from build123d import *

# Parameters (mm, degrees)
F0_W     = 80
F0_H     = 80
F1_DEPTH = 10
F2_SIZE2 = 9.99999
F2_SIZE  = 9.99999
F3_W     = 10
F3_H     = 40
F4_DEPTH = 10
F6_DEPTH = 8


# Not quite as in the source:
# - a fillet or chamfer is up to 0.001 mm smaller than in the source, because OpenCascade refuses the exact size


with BuildPart() as f1:
    # F0 (on Top) → F1 (new body)
    with BuildSketch(Plane.XY):
        Rectangle(F0_W, F0_H)
    extrude(amount=F1_DEPTH)

    # F2 (size 10 and 10 in the source; OpenCascade refuses exactly that, so slightly less here)
    f2_edges = [f1.edges().sort_by_distance(p)[0] for p in [
        (0, 40, 10),
        (-40, 0, 10),
        (0, -40, 10),
        (40, 0, 10),
    ]]
    chamfer(f2_edges, length=F2_SIZE, length2=F2_SIZE2)

    # F3 (on face) → F4 (join)
    with BuildSketch(Plane.XY.offset(10)):
        with Locations((25, 0)):
            Rectangle(F3_W, F3_H)
        with Locations((-25, 0)):
            Rectangle(F3_W, F3_H)
    extrude(amount=F4_DEPTH)

    # F5 (on face) → F6 (cut)
    with BuildSketch(Plane.XY.offset(10)):
        with BuildLine():
            Line((-3.8890872965, -3.8890872965), (-10.2530483272, -10.2530483272))
            ThreePointArc((-10.2530483272, -10.2530483272), (-5.3489923662, -11.2285257082), (-2.5710678119, -7.0710678119))
            ThreePointArc((-2.5710678119, -7.0710678119), (-2.9136099156, -5.3489923662), (-3.8890872965, -3.8890872965))
        make_face()
        with BuildLine():
            Line((3.8890872965, 3.8890872965), (10.2530483272, 10.2530483272))
            ThreePointArc((10.2530483272, 10.2530483272), (3.8890872965, 10.2530483272), (3.8890872965, 3.8890872965))
        make_face()
        with BuildLine():
            ThreePointArc((-2.5710678119, 7.0710678119), (-5.3489923662, 11.2285257082), (-10.2530483272, 10.2530483272))
            Line((-10.2530483272, 10.2530483272), (-3.8890872965, 3.8890872965))
            ThreePointArc((-3.8890872965, 3.8890872965), (-2.9136099156, 5.3489923662), (-2.5710678119, 7.0710678119))
        make_face()
        with BuildLine():
            ThreePointArc((11.5710678119, 7.0710678119), (11.2285257082, 8.7931432575), (10.2530483272, 10.2530483272))
            Line((10.2530483272, 10.2530483272), (3.8890872965, 3.8890872965))
            ThreePointArc((3.8890872965, 3.8890872965), (8.7931432575, 2.9136099156), (11.5710678119, 7.0710678119))
        make_face()
        with BuildLine():
            ThreePointArc((3.8890872965, -3.8890872965), (3.8890872965, -10.2530483272), (10.2530483272, -10.2530483272))
            Line((10.2530483272, -10.2530483272), (3.8890872965, -3.8890872965))
        make_face()
        with BuildLine():
            Line((-3.8890872965, 3.8890872965), (-10.2530483272, 10.2530483272))
            ThreePointArc((-10.2530483272, 10.2530483272), (-10.2530483272, 3.8890872965), (-3.8890872965, 3.8890872965))
        make_face()
        with BuildLine():
            ThreePointArc((-3.8890872965, -3.8890872965), (-10.2530483272, -3.8890872965), (-10.2530483272, -10.2530483272))
            Line((-10.2530483272, -10.2530483272), (-3.8890872965, -3.8890872965))
        make_face()
        with BuildLine():
            Line((3.8890872965, -3.8890872965), (10.2530483272, -10.2530483272))
            ThreePointArc((10.2530483272, -10.2530483272), (11.2285257082, -8.7931432575), (11.5710678119, -7.0710678119))
            ThreePointArc((11.5710678119, -7.0710678119), (8.7931432575, -2.9136099156), (3.8890872965, -3.8890872965))
        make_face()
    extrude(amount=-F6_DEPTH, mode=Mode.SUBTRACT)


solid = f1.part
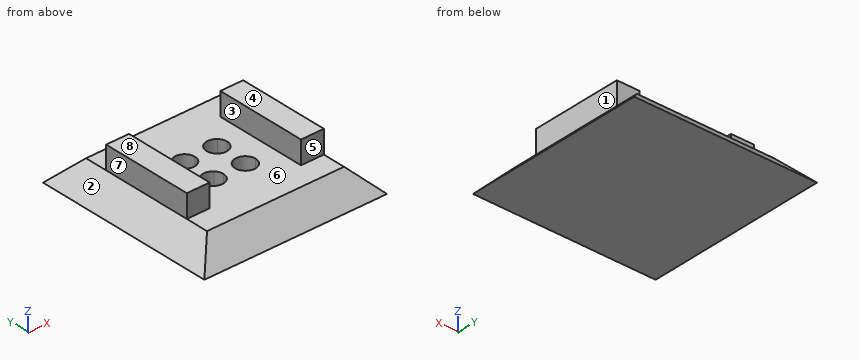
The listing builds one solid part. Answer for the finished solid, in the listing's coordinates (mm). Face numbers are marked on the shaded views. A direction names the side the tool comes from. Coordinates: 2 decimals unless noted, no trailing zeros. Order: outer loops, then holes, each group sorted by start corner. A loop starts at its lowest first (then second) coordinate and runs counter-clockwise, first axis right, second up. Notation, with made-up numbers: (62.25, 85) -> (78.25, 85) arc R27 ccw to (78.25, 114) -> close; hole circle Ø11 at (74.25, -29.5). An arc over 180 degrees is marked (long way). Answer in a Markdown table with one row per item. Add a question column.
Item 1: Determine the mould class of the marked faces 6, 7 and 8 for opening direction X: +X half, -X half, draft (parallel to the pull), parting line (faces both ways), or undercut.
Item 2: Find the intervals of material crossed by L1, parallel to X at y = -13, z = 10.75; L2, parallel to Z at x = -20, y = 20.5; L3, parallel to Z at x = -6, y = -7.5, in increasing order. Write a range as from..to.
Item 3: Find section D-D (z = 3.5). Write down the section's boundary in (x, y).
Item 4: Find section A-A (z = 13.5). Write down the section's boundary in (x, y).
Item 5: Each of these flat-tipped pins is pushed along its axis until it touches: P1, Ø3, axis at y = 15, z = 7.5, coming from the -X side; P2, Ø11, axis at x = -24, z = 13, coming from the -Y side; P3, Ø3, axis at y = 2, z = 15, coming from the -X side. Where does it stop, or does it pass through?
Item 6: Which of the six approach directions +Z, -Z, +X, -X, +Y, -Y give full straight-line access (tool end or side, diameter ignored) to the marked faces 1, 2, 3, 4 and 5?
Result set:
| question | item | result |
|---|---|---|
| 1 | face 6 | undercut |
| 1 | face 7 | -X half |
| 1 | face 8 | draft |
| 2 | L1 | x = -30..-20, 20..30 |
| 2 | L2 | z = 0..10 |
| 2 | L3 | z = 0..2 |
| 3 | outline | (-36.5, -36.5) -> (36.5, -36.5) -> (36.5, 36.5) -> (-36.5, 36.5) -> close; hole circle Ø9 at (-7.07, -7.07); hole circle Ø9 at (-7.07, 7.07); hole circle Ø9 at (7.07, -7.07); hole circle Ø9 at (7.07, 7.07) |
| 4 | outline | (-30, -20) -> (-20, -20) -> (-20, 20) -> (-30, 20) -> close; (20, -20) -> (30, -20) -> (30, 20) -> (20, 20) -> close |
| 5 | P1 | stops at x = -34 |
| 5 | P2 | stops at y = -32.5 |
| 5 | P3 | stops at x = -30 |
| 6 | face 1 | +Z, +X, +Y, -Y |
| 6 | face 2 | +Z, -X, +Y, -Y |
| 6 | face 3 | +Z, +Y, -Y |
| 6 | face 4 | +Z, +X, -X, +Y, -Y |
| 6 | face 5 | +Z, +X, -X, -Y |
